Part print with two shaded views. Sizes in mm from the minimum x, y, z corner. A direction names the side the tool comes from. Coordinates: 2 decimals unless noted, no trailing zeros. Loops run counter-clockwise (first coordinate to the right, second up) from the corner with the lowest first, then second, coordinate; pieces in that order, holes last. Notation, with made-up numbers: (-2, 66.5) -> (25, 66.5) arc R17 cw to (25, 90.5) -> close; hole circle Ø1 at (68.25, 18). An arc over 180 degrees is marked (long way). One line per item, written item: value. Start each with the question number.
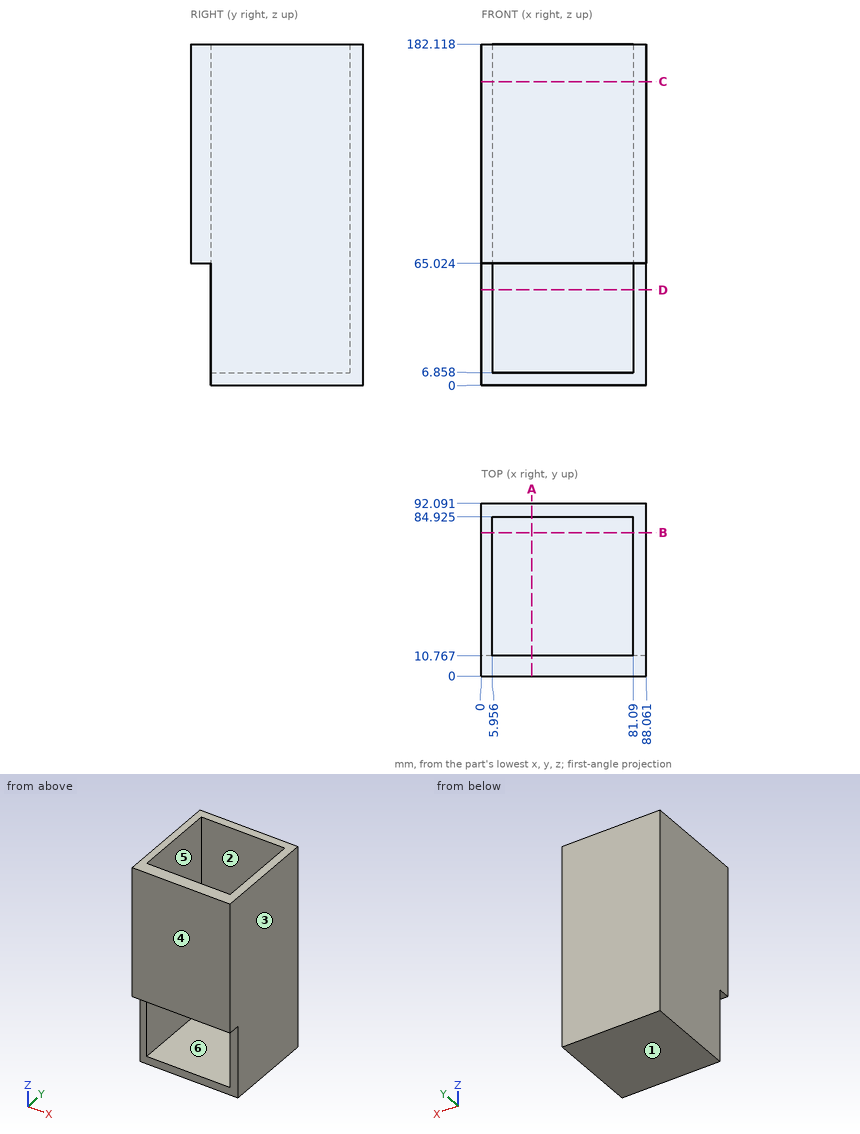
Item 1: Band-saw the part on B-B, the plane y = 76.5. List the corners of the cut face in (x, z) (1 decimal), and give its area (3 significant figures).
Item 2: Drop flat-ended pins along their axis: pin 1 Ø5.5 at (x, y) = (42.5, 6) entering from -Z; pin 2 Ø1 at (x, z) = (71.5, 48) entering from -Y (1 decimal). Give the stop position or say it passes through.
Item 3: Band-saw the part on C-C, the plane z = 162. List the corners of the cut face in (x, y) (1 decimal), and give its area (3 significant figures).
Item 4: Band-saw the part on D-D, the plane z = 51. List the corners of the cut face in (x, y) (1 decimal), and give its area (3 significant figures).
Item 5: Two-plate mould, pull along X, no slides. Class the marked faces 1, 2 and 3: +X half, -X half, draft (parallel to the pull), parting line (faces both ways), or undercut.
Item 6: Band-saw the part on A-A, the plane x = 27. List the corners of the cut face in (y, z) (1 decimal).
Item 7: Tool access for the marked faces 4, 5 and 6: list every direction of +Z, -Z, +X, -X, +Y, -Y with a clear straight run to the whole face (end or side of a thin tool).
Item 8: Probe probe 1 along X at (y, z) = (48.5, 101) (1 decimal); probe 2 along Y at (x, z) = (76.5, 84) (1 decimal); probe 3 along Z at (x, y) = (61.5, 56). List the from-to ranges inside material, lowest first.
Worked out:
1. outline: (0, 0) -> (88.1, 0) -> (88.1, 182.1) -> (81.1, 182.1) -> (81.1, 6.9) -> (6, 6.9) -> (6, 182.1) -> (0, 182.1) -> close
1. area: 2,870 mm²
2. pin 1: stops at z = 65.02
2. pin 2: stops at y = 84.9
3. outline: (0, 0) -> (88.1, 0) -> (88.1, 92.1) -> (0, 92.1) -> close; hole (6, 10.8) -> (81.1, 10.8) -> (81.1, 84.9) -> (6, 84.9) -> close
3. area: 2,540 mm²
4. outline: (0, 10.8) -> (6, 10.8) -> (6, 84.9) -> (81.1, 84.9) -> (81.1, 10.8) -> (88.1, 10.8) -> (88.1, 92.1) -> (0, 92.1) -> close
4. area: 1,590 mm²
5. face 1: draft
5. face 2: undercut
5. face 3: +X half
6. outline: (0, 65) -> (10.8, 65) -> (10.8, 182.1) -> (0, 182.1) -> close; (10.8, 0) -> (92.1, 0) -> (92.1, 182.1) -> (84.9, 182.1) -> (84.9, 6.9) -> (10.8, 6.9) -> close
7. face 4: +Z, -Z, +X, -X, -Y
7. face 5: +Z
7. face 6: +Z, -Y
8. probe 1: x = 0 to 6, 81.1 to 88.1
8. probe 2: y = 0 to 10.8, 84.9 to 92.1
8. probe 3: z = 0 to 6.86
